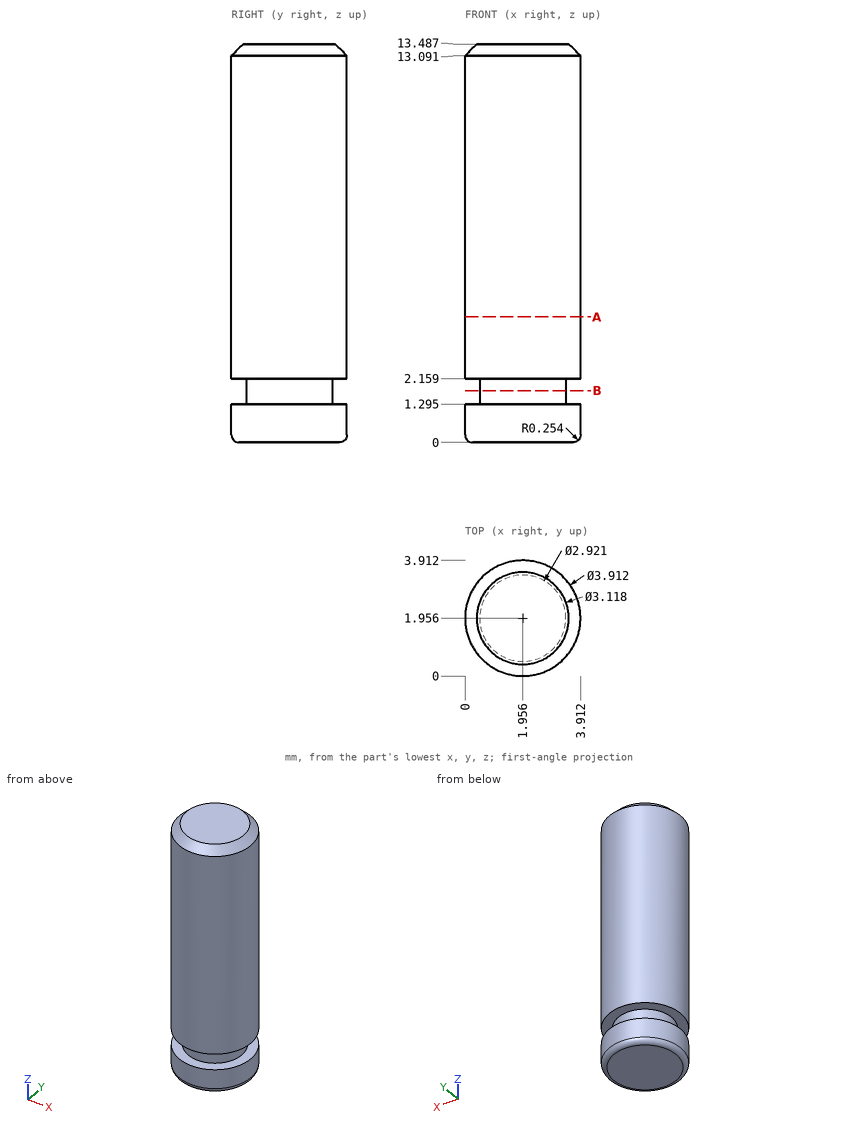
Study the drawing (mm; zero at the part's minimum x, y, z) and answer. Round coordinates to 2 decimals unless told otherwise and drop trailing zeros. Loops run counter-clockwise (first coordinate to the right, second up) from the corner with the lowest first, then second, coordinate; pieces in that order, holes last. Notation, with made-up numbers: M 11,51.25 L 45,51.25 A30 cw 45,86.25 Z; hole C 73,-14 d5. An arc over 180 degrees is marked long. One line per question, with ' | ' between items.
Q1. Find section B-B, the plane z = 1.75. Give the vertices of the cut face in (x, y) (1 decimal).
Conclusion:
outline: C 2,2 d2.9
Q2. Consider line 1 along Z through (x, y) = (1, 3.1) (1 decimal); line 2 along Y through (x, z) = (2, 1.5) (1 decimal); line 3 along X through (y, z) = (0.5, 9.75). Determine where each line is inside the solid, lowest interval first. Write a range as from..to.
Conclusion:
line 1: z = 0..1.3, 2.2..13.5 | line 2: y = 0.5..3.4 | line 3: x = 0.65..3.26
Q3. Find section A-A, the plane z = 4.25. Give the vertices of the cut face in (x, y) (1 decimal).
Conclusion:
outline: C 2,2 d3.9
Q4. This flat-tipped pin is pushed along its axis until it touches: pin 1 Ø2 at (x, z) = (2.5, 5) entering from +Y. Where does it stop, or does it pass through?
Conclusion:
pin 1: stops at y = 3.91
